from build123d import *

# Parameters (mm, degrees)
F0_W     = 45
F0_H     = 70
F1_DEPTH = 25
F3_DEPTH = 20
F5_DEPTH = 25
F7_DEPTH = 40


with BuildPart() as f1:
    # F0 (on Top) → F1 (new body)
    with BuildSketch(Plane.XY):
        with Locations((-1.3771308213, -35)):
            Rectangle(F0_W, F0_H)
    extrude(amount=F1_DEPTH)

    # F2 (on face) → F3 (cut)
    with BuildSketch(Plane.XY.offset(25)):
        with BuildLine():
            Line((-1.3771308213, -32.347425729), (-1.3771308213, -65.347425729))
            ThreePointArc((-1.3771308213, -65.347425729), (10.2901310682, -60.5146876186), (15.1228691787, -48.847425729))
            ThreePointArc((15.1228691787, -48.847425729), (10.2901310682, -37.1801638395), (-1.3771308213, -32.347425729))
        make_face()
        with BuildLine():
            ThreePointArc((-1.3771308213, -32.347425729), (-17.8771308213, -48.847425729), (-1.3771308213, -65.347425729))
            Line((-1.3771308213, -65.347425729), (-1.3771308213, -32.347425729))
        make_face()
    extrude(amount=-F3_DEPTH, mode=Mode.SUBTRACT)

    # F4 (on face) → F5 (join)
    with BuildSketch(Plane.XY.offset(25)):
        Polygon((-23.8771308213, 0), (-23.8771308213, -27.1776393056), (0, -27.1776393056), (21.1228691787, -27.1776393056), (21.1228691787, 0), align=None)
    extrude(amount=F5_DEPTH)

    # F6 (on face) → F7 (cut)
    with BuildSketch(Plane.XY.offset(50)):
        with BuildLine():
            ThreePointArc((-0.1445451178, -2.8525939696), (-8.0951260785, -5.7974552618), (-11.4385654107, -13.5888196528))
            Line((-11.4385654107, -13.5888196528), (-0.6885654107, -13.5888196528))
            Line((-0.6885654107, -13.5888196528), (-0.1445451178, -2.8525939696))
        make_face()
        with BuildLine():
            Line((-0.6885654107, -13.5888196528), (-11.4385654107, -13.5888196528))
            ThreePointArc((-11.4385654107, -13.5888196528), (-8.4799298017, -20.9953803206), (-1.2325857035, -24.325045336))
            Line((-1.2325857035, -24.325045336), (-0.6885654107, -13.5888196528))
        make_face()
        with BuildLine():
            Line((-0.1445451178, -2.8525939696), (-0.6885654107, -13.5888196528))
            Line((-0.6885654107, -13.5888196528), (10.0614345893, -13.5888196528))
            ThreePointArc((10.0614345893, -13.5888196528), (7.1027989804, -6.182258985), (-0.1445451178, -2.8525939696))
        make_face()
        with BuildLine():
            Line((10.0614345893, -13.5888196528), (-0.6885654107, -13.5888196528))
            Line((-0.6885654107, -13.5888196528), (-1.2325857035, -24.325045336))
            ThreePointArc((-1.2325857035, -24.325045336), (6.7179952571, -21.3801840438), (10.0614345893, -13.5888196528))
        make_face()
    extrude(amount=-F7_DEPTH, mode=Mode.SUBTRACT)


solid = f1.part
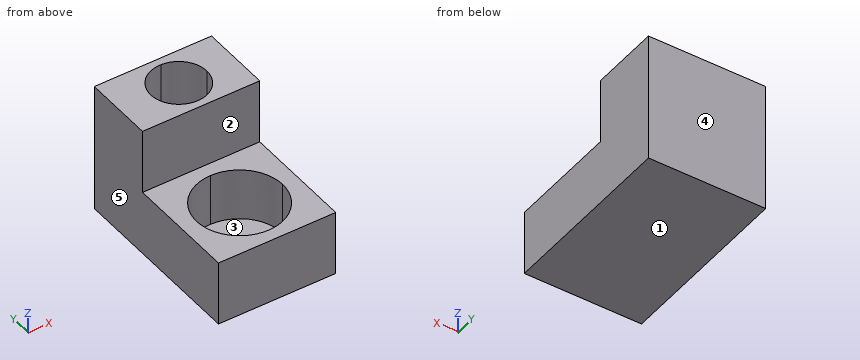
Can you work these out from the model? Positions are in its coordinate system, mm. Face numbers are marked on the shaded views. A direction names the side the tool comes from. Coordinates: 2 decimals unless noted, no trailing zeros. Write each loop counter-clockwise with the first axis right and the second up, starting at its lowest first coordinate (ties: lowest second). Pieces come first, ordered by that corner, then holes. Notation, with made-up numbers: (62.5, 72) -> (69.5, 72) arc R22 cw to (69.5, 109) -> close; hole circle Ø5 at (18.5, 88.25). An arc over 180 degrees is marked (long way). Answer as CSV lines item,"result".
1) If we section it at B-B on z = 44: Please give me the cut outline in (x, y), then the cut area to 3 significant figures.
Check result:
outline,"(-23.88, -27.18) -> (21.12, -27.18) -> (21.12, 0) -> (-23.88, 0) -> close; hole circle Ø21.5 at (-0.69, -13.59)"
area,"860 mm²"
2) On a 3-axis mill with a long thin cutter (end or side, diameter ignored), from which of +Z, -Z, +X, -X, +Y, -Y can I reach the whole of each face in a straight line? I mean the marked faces 1 and 2. Say none if no direction works.
Check result:
face 1,"-Z, +X, -X, +Y, -Y"
face 2,"+Z, +X, -X, -Y"
3) If I drill on line 1 (Y direction, x = -1, z = 29); line 2 (Z direction, x = 2, y = -9.5); line 3 (Z direction, x = -8, y = -61.5), over which ranges is the centre line in solid material (lowest first)? Write a range as from..to.
Check result:
line 1,"-27.18..-24.33, -2.84..0"
line 2,"0..10"
line 3,"0..5"
4) If we section it at C-C on x = 18.5: Please give me the cut outline in (y, z).
Check result:
outline,"(-70, 0) -> (0, 0) -> (0, 50) -> (-27.18, 50) -> (-27.18, 25) -> (-70, 25) -> close"
5) If we section it at D-D on y = -41: Please give me the cut outline in (x, z).
Check result:
outline,"(-23.88, 0) -> (21.12, 0) -> (21.12, 25) -> (13.14, 25) -> (13.14, 5) -> (-15.89, 5) -> (-15.89, 25) -> (-23.88, 25) -> close"
6) If we section it at A-A on z = 14: Please give me the cut outline in (x, y), then the cut area to 3 significant figures.
Check result:
outline,"(-23.88, -70) -> (21.12, -70) -> (21.12, 0) -> (-23.88, 0) -> close; hole circle Ø33 at (-1.38, -48.85); hole circle Ø21.5 at (-0.69, -13.59)"
area,"1,930 mm²"
7) Will these pins go through, and if not, where does the flat tip stop? P1, Ø16.5, axis at x = -9, y = -48, coming from the +Z side; P2, Ø6.5, axis at x = -2.5, y = -10.5, coming from the +Z side; P3, Ø6, axis at x = -14, z = 33.5, coming from the -Y side.
Check result:
P1,"z = 5"
P2,"z = 10"
P3,"y = -27.18"
8) If we mould it in two halves opening along X, with no side actions, what happens to the marked faces 3, 4 and 5? For each: +X half, -X half, draft (parallel to the pull), parting line (faces both ways), or undercut.
Check result:
face 3,"undercut"
face 4,"draft"
face 5,"-X half"
